Autodesk Inventor part; units mm, degrees
ref_plane "YZ Plane" through (0, 0, 0) normal (1, 0, 0) x (0, 1, 0)
ref_plane "XZ Plane" through (0, 0, 0) normal (0, 1, 0) x (-1, 0, 0)
ref_plane "XY Plane" through (0, 0, 0) normal (0, 0, 1) x (1, 0, 0)
sketch "Sketch1" plane through (0, 0, 0) normal (0, 0, 1) x (1, 0, 0)
  line L0 (0, 0) -> (0, 71) construction
  circle A0 centre (0, 63.5) radius 7.5 construction
  circle A1 centre (0, 7.5) radius 7.5 construction
  line L1 (7.5, 63.5) -> (7.5, 7.5)
  line L2 (-7.5, 7.5) -> (-7.5, 63.5)
  arc A2 (7.5, 63.5) -> (-7.5, 63.5) centre (0, 63.5) ccw
  arc A3 (-7.5, 7.5) -> (7.5, 7.5) centre (0, 7.5) ccw
  circle A4 centre (0, 35.5) radius 3.9
  circle A5 centre (0, 63.5) radius 3.75
  circle A6 centre (0, 7.5) radius 3.75
  dimension "d1" = 15
  dimension "d2" = 15
  dimension "d3" = 7.8
  dimension "d4" = 7.5
  dimension "d5" = 7.5
  dimension "d21" = 56
extrude "Extrusion1" add sketch "Sketch1" along normal blind 3
sketch "Sketch3" plane through (0, 0, 0) normal (0, 0, -1) x (-1, 0, 0)
  circle A0 centre (0, 63.5) radius 3.75
  circle A1 centre (0, 7.5) radius 3.75
  point P0 (0, 0)
extrude "Extrusion2" add sketch "Sketch3" against normal blind 12
sketch "Sketch4" plane through (0, 63.5, 12) normal (0, 0, 1) x (1, 0, 0)
  circle A0 centre (0, 0) radius 3.75
  circle A1 centre (0, -56) radius 3.75
  circle A2 centre (0, 0) radius 1.5
  circle A3 centre (0, -56) radius 1.5
  point P0 (0, -63.5)
  dimension "d10" = 3
  dimension "d11" = 3
extrude "Extrusion3" cut sketch "Sketch4" against normal through all contours A2 | A3
sketch "Sketch5" plane through (0, 0, 3) normal (0, 0, 1) x (1, 0, 0)
  circle A0 centre (0, 63.5) radius 1.5
  line L0 (7.5, 43) -> (7.5, 28)
  line L1 (-7.5, 43) -> (-7.5, 28)
  circle A1 centre (0, 35.5) radius 3.9
  line L2 (-7.5, 43) -> (7.5, 43)
  line L3 (-7.5, 28) -> (7.5, 28)
  point P0 (0, 0)
  point P1 (-7.5, 35.5)
  point P2 (7.5, 35.5)
  point P3 (7.5, 63.5)
  point P4 (-7.5, 63.5)
  point P5 (7.5, 7.5)
  dimension "d22" = 15
extrude "Extrusion4" add sketch "Sketch5" along normal blind 9 contours L0 L3 L1 L2
sketch "Sketch6" plane through (0, 0, 0) normal (1, 0, 0) x (0, 1, 0)
  line L0 (7.5, 0) -> (63.5, 0)
  line L1 (7.5, 0) -> (7.5, 3)
  line L2 (63.5, 3) -> (43, 3)
  line L3 (28, 3) -> (28, 12)
  line L4 (43, 12) -> (28, 12)
  line L5 (43, 3) -> (43, 12)
  line L6 (63.5, 0) -> (63.5, 3)
  circle A0 centre (35.5, 7.5) radius 1.5
  line L7 (28, 3) -> (7.5, 3)
  point P0 (0, 0)
  point P1 (35.5, 12)
  point P2 (43, 7.5)
  dimension "d18" = 3
extrude "Extrusion5" cut sketch "Sketch6" against normal through all contours A0
properties part number "WaveGenerator" material "ABS Plastic"
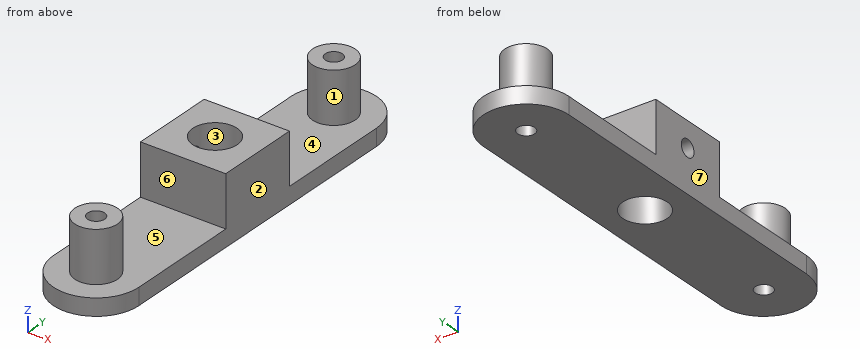
Geometry: final body of the model. Coordinates: model frame, mm. Face numbers are marked on the shaded views. A direction names the side the tool comes from. Coordinates: 2 decimals unless noted, no trailing zeros. Order: outer loops, then holes, each group sorted by start corner. A loop starts at its lowest first (then second) coordinate and runs counter-clockwise, first axis right, second up.
Item 1: Section query B-B (z = 7.5). Output: boundary loops of the cut face in (x, y).
Answer:
outline: (-7.5, 28) - (7.5, 28) - (7.5, 43) - (-7.5, 43) - (-7.5, 37) - (-3.6, 37) arc R3.9 cw (long way) to (-3.6, 34) - (-7.5, 34) - close; circle Ø7.5 at (0, 7.5); circle Ø7.5 at (0, 63.5); hole circle Ø3 at (0, 7.5); hole circle Ø3 at (0, 63.5)
Item 2: Draft query along X for the marked faces 1, 2, 3 and 4. Return one class per face: released by +X, released by -X, zero draft, split by the parting line, or undercut.
Answer:
face 1: split by the parting line
face 2: released by +X
face 3: undercut
face 4: zero draft
Item 3: Section query A-A (z = 11.25). Output: boundary loops of the cut face in (x, y), then the cut area to 3 significant figures.
Answer:
outline: (-7.5, 28) - (7.5, 28) - (7.5, 43) - (-7.5, 43) - close; circle Ø7.5 at (0, 7.5); circle Ø7.5 at (0, 63.5); hole circle Ø7.8 at (0, 35.5); hole circle Ø3 at (0, 7.5); hole circle Ø3 at (0, 63.5)
area: 251 mm2
Item 4: Access query for the marked faces 5, 6 and 7. Directions: +Z, -Z, +X, -X, +Y, -Y. A direction counts if a zero-diameter tool reaches every point of the face in a straight line with its end or side. Return the directions, or none.
Answer:
face 5: +Z
face 6: +Z, +X, -X
face 7: +Z, -Z, -X, +Y, -Y
Item 5: Material intervals for line 1 along Y through (x, z) = (0, 5.5); line 2 along Y through (x, z) = (0, 2.5); line 3 along Y through (x, z) = (-0.75, 6), sorted ascending.
Answer:
line 1: y = 3.75 to 6, 9 to 11.25, 28 to 31.6, 39.4 to 43, 59.75 to 62, 65 to 67.25
line 2: y = 0 to 6, 9 to 31.6, 39.4 to 62, 65 to 71
line 3: y = 3.83 to 6.2, 8.8 to 11.17, 28 to 31.67, 39.33 to 43, 59.83 to 62.2, 64.8 to 67.17
Item 6: Section query C-C (y = 35.5). Output: boundary loops of the cut face in (x, z), then the cut area to 3 significant figures.
Answer:
outline: (-7.5, 0) - (-3.9, 0) - (-3.9, 6) - (-7.5, 6) - close; (-7.5, 9) - (-3.9, 9) - (-3.9, 12) - (-7.5, 12) - close; (3.9, 0) - (7.5, 0) - (7.5, 12) - (3.9, 12) - close
area: 75.6 mm2
Item 7: Section query D-D (x = 0). Output: boundary loops of the cut face in (y, z).
Answer:
outline: (0, 0) - (6, 0) - (6, 12) - (3.75, 12) - (3.75, 3) - (0, 3) - close; (9, 0) - (31.6, 0) - (31.6, 12) - (28, 12) - (28, 3) - (11.25, 3) - (11.25, 12) - (9, 12) - close; (39.4, 0) - (62, 0) - (62, 12) - (59.75, 12) - (59.75, 3) - (43, 3) - (43, 12) - (39.4, 12) - close; (65, 0) - (71, 0) - (71, 3) - (67.25, 3) - (67.25, 12) - (65, 12) - close
Item 8: Contact query for flat-ended pins moving along their axis: P1, Ø2.5, axis at x = 1, z = 7, coming from the +Y side; P2, Ø8, axis at x = -4.5, y = 57, coming from the +Z side; P3, Ø2, axis at x = -4, z = 3, coming from the -Y side. Output: stop coordinate, or through.
Answer:
P1: stops at y = 67.25
P2: stops at z = 3
P3: stops at y = 0.63
